CAD build for the part. Positions are in the model's coordinates, mm. Face numbers are marked on the shaded views. A direction names the side the tool comes from. Coordinates: 2 decimals unless noted, no trailing zeros. Order: outer loops, then holes, each group sorted by start corner. A loop starts at its lowest first (then second) coordinate and runs counter-clockwise, first axis right, second up. Notation, with made-up numbers: (65, 33.25) - (96, 33.25) arc R12 cw to (96, 41.25) - close; hole circle Ø1 at (6, -4). An arc over 180 degrees is marked (long way). Use one line per item in the form item = value.
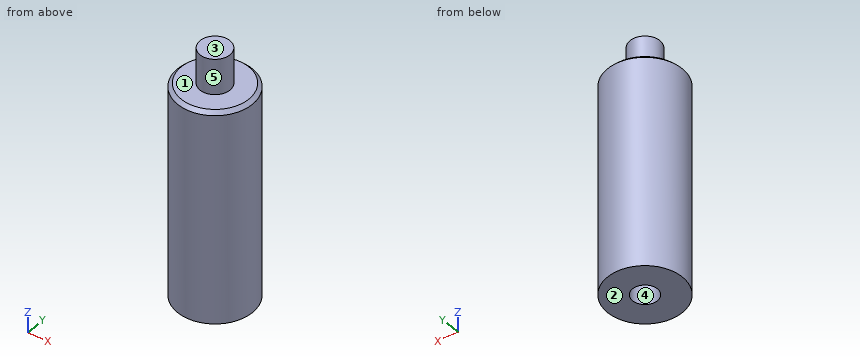
```python
from build123d import *

# Parameters (mm, degrees)
ESQUISSE1_R                  = 5.25
BOSS_EXTRU_1_DEPTH           = 30
CHANFREIN1_SIZE              = 0.5
ESQUISSE2_R                  = 1.75
ENL_V_MAT_EXTRU_1_DEPTH      = 1
ENL_V_MAT_EXTRU_1_DEPTH_BACK = 15
ESQUISSE4_R                  = 2.1
BOSS_EXTRU_2_DEPTH           = 5


with BuildPart() as part:
    # Esquisse1 → Boss.-Extru.1 (new body)
    with BuildSketch(Plane.XY):
        Circle(ESQUISSE1_R)
    extrude(amount=BOSS_EXTRU_1_DEPTH)

    # Chanfrein1
    chanfrein1_edges = [part.edges().sort_by_distance(p)[0] for p in [
        (-5.25, 0, 30),
    ]]
    chamfer(chanfrein1_edges, length=CHANFREIN1_SIZE)

    # Esquisse2 → Enlèv. mat.-Extru.1 (cut, two sides)
    with BuildSketch(Plane(origin=(0, 0, 0), x_dir=(-1, 0, 0), z_dir=(0, 0, -1))) as enl_v_mat_extru_1_sk:
        Circle(ESQUISSE2_R)
    extrude(amount=ENL_V_MAT_EXTRU_1_DEPTH, mode=Mode.SUBTRACT)
    extrude(enl_v_mat_extru_1_sk.sketch, amount=-ENL_V_MAT_EXTRU_1_DEPTH_BACK, mode=Mode.SUBTRACT)

    # Esquisse4 → Boss.-Extru.2 (add)
    with BuildSketch(Plane.XY.offset(30)):
        Circle(ESQUISSE4_R)
    extrude(amount=BOSS_EXTRU_2_DEPTH)


solid = part.part
```
Item 1: Drill centre lines: line 1 (Y direction, x = 0, z = 9.5); line 2 (Z direction, x = 2.25, y = -0.75); line 3 (X direction, y = -0.5, z = 14). Where is each one in solid material? Low to high. Write a range as [from, to].
Derived:
line_1 = [-5.25, -1.75], [1.75, 5.25]
line_2 = [0, 30]
line_3 = [-5.23, -1.68], [1.68, 5.23]
Item 2: Two-plate mould, pull along X, no slides. Class the marked faces 3, 4 and 5: +X half, -X half, draft (parallel to the pull), parting line (faces both ways), or undercut.
Derived:
face_3 = draft
face_4 = undercut
face_5 = parting line
Item 3: Drop flat-ended pins along their axis: pin 1 (3 mm diameter, centred on x = 0, y = 0, fed in from -Z); pin 2 (4.5 mm diameter, centred on x = 0, y = 0, fed in from -Z); pin 3 (1 mm diameter, centred on y = 4, z = 10, fed in from +X); pin 4 (4 mm diameter, centred on y = 4, z = 13.5, fed in from -X). Give the stop position or say it passes through.
Derived:
pin_1 = 15
pin_2 = 0
pin_3 = 3.91
pin_4 = -4.85
Item 4: Cut at C-C, the plane z = 29. Write the cut outline in (x, y), plus the area to 3 significant figures.
Derived:
outline = circle Ø10.5 at (0, 0)
area = 86.6 mm²
Item 5: 3-axis set-ups, long thin cutter, end or side, ignore diameter. For the marked faces 1 and 2: which of +Z, -Z, +X, -X, +Y, -Y reach the whole face in a straight line?
Derived:
face_1 = +Z
face_2 = -Z, +X, -X, +Y, -Y
Item 6: Cut at A-A, the plane y = 0. Write the cut outline in (x, z).
Derived:
outline = (-5.25, 0) - (-1.75, 0) - (-1.75, 15) - (1.75, 15) - (1.75, 0) - (5.25, 0) - (5.25, 29.5) - (4.75, 30) - (2.1, 30) - (2.1, 35) - (-2.1, 35) - (-2.1, 30) - (-4.75, 30) - (-5.25, 29.5) - close
